The figure shows three views and two pictorial views of one solid part (mm, origin at its lowest corner). Answer the questions. A direction names the side the tool comes from. Coordinates: 2 decimals unless noted, no trailing zeros. Write each loop counter-clockwise with the first axis right and the second up, starting at its lowest first coordinate (ties: lowest second). Pieces come first, ordered by that corner, then holes. Notation, with made-up numbers: (0.25, 51.5) - (35.25, 51.5) arc R21 cw to (35.25, 88.5) - close; hole circle Ø9 at (19.25, -27). An arc over 180 degrees is marked (long way). Use a Markdown table: item, result. Add a question column.
(1) The part is cut by section C-C, the plane z = 1.25. State how many separate pieces and enclosed holes the cut face has, then the cut area to 3 significant figures.
(2) The part is cut by section B-B, the plane y = 5. Give the vertices of the cut face in (x, z), then the cut area to 3 significant figures.
(3) Find the intervals of material crossed by line 1 (Y direction, x = 48, z = 2.75); line 2 (X direction, y = 45, z = 2.35); line 3 (X direction, y = 26.5, z = 1.75), in increasing order. Write a range as from..to.
(4) The part is cut by section D-D, the plane x = 48. Give the vertices of the cut face in (y, z), then the cut area to 3 significant figures.
(5) A tool of negligible diameter and unlimited length cuts with its end or side. For the marked faces 1 and 2, from which of +Z, -Z, +X, -X, +Y, -Y can it reach the whole face along a straight path? Write none if from no direction.
(6) Given pin 1 Ø2 at (y, z) = (10, 7) entering from -X; pin 2 Ø3 at (y, z) = (34.5, 7) entering from -X; pin 3 Ø1.8 at (y, z) = (45.5, 7) entering from +X, each flat-ended and moving along its own axis, determine where each tip first touches the part or whether it passes through.
(7) The part is cut by section A-A, the plane x = 23.5. Give the vertices of the cut face in (y, z).
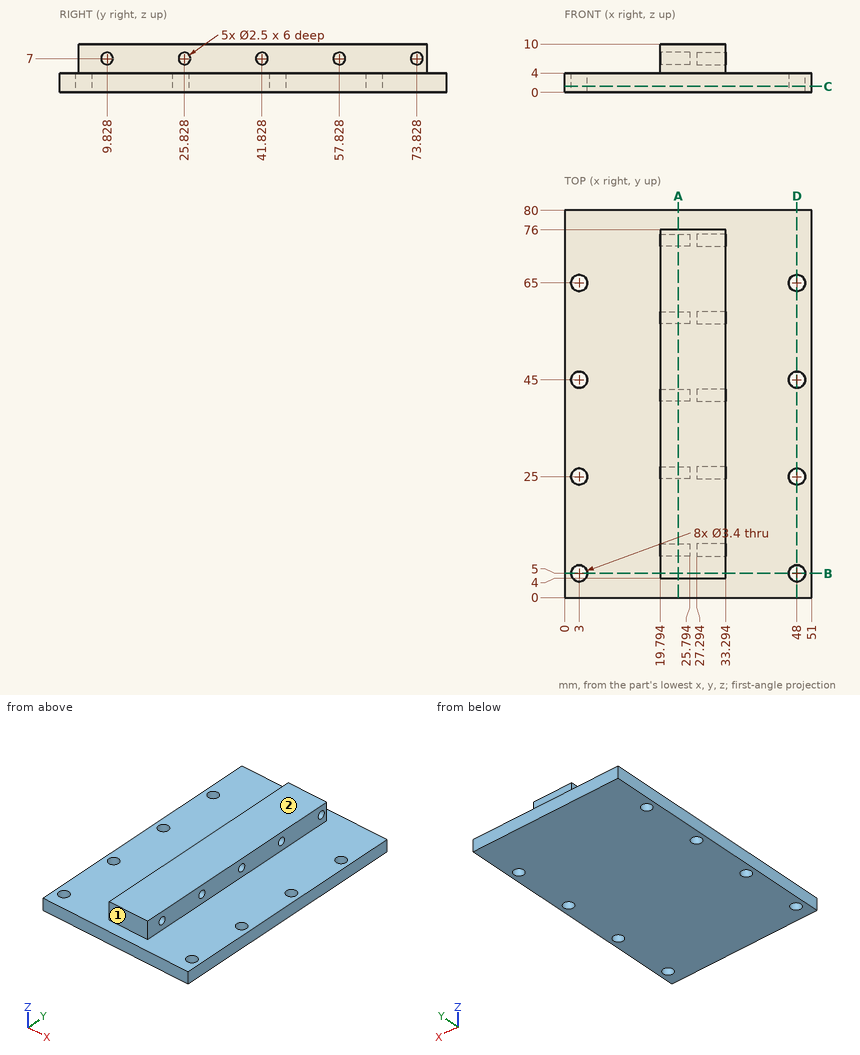
Model answer:
| question | item | result |
|---|---|---|
| 1 | separate pieces | 1 |
| 1 | enclosed holes | 8 |
| 1 | area | 4,010 mm^2 |
| 2 | outline | (0, 0) - (1.3, 0) - (1.3, 4) - (0, 4) - close; (4.7, 0) - (46.3, 0) - (46.3, 4) - (33.29, 4) - (33.29, 10) - (19.79, 10) - (19.79, 4) - (4.7, 4) - close; (49.7, 0) - (51, 0) - (51, 4) - (49.7, 4) - close |
| 2 | area | 258 mm^2 |
| 3 | line 1 | 0..3.3, 6.7..23.3, 26.7..43.3, 46.7..63.3, 66.7..80 |
| 3 | line 2 | 0..1.3, 4.7..46.3, 49.7..51 |
| 3 | line 3 | 0..2.2, 3.8..47.2, 48.8..51 |
| 4 | outline | (0, 0) - (3.3, 0) - (3.3, 4) - (0, 4) - close; (6.7, 0) - (23.3, 0) - (23.3, 4) - (6.7, 4) - close; (26.7, 0) - (43.3, 0) - (43.3, 4) - (26.7, 4) - close; (46.7, 0) - (63.3, 0) - (63.3, 4) - (46.7, 4) - close; (66.7, 0) - (80, 0) - (80, 4) - (66.7, 4) - close |
| 4 | area | 266 mm^2 |
| 5 | face 1 | +Z, +X, -X, -Y |
| 5 | face 2 | +Z, +X, -X, +Y, -Y |
| 6 | pin 1 | x = 25.79 |
| 6 | pin 2 | x = 19.79 |
| 6 | pin 3 | x = 33.29 |
| 7 | outline | (0, 0) - (80, 0) - (80, 4) - (76, 4) - (76, 10) - (4, 10) - (4, 4) - (0, 4) - close; hole circle Ø2.5 at (9.83, 7); hole circle Ø2.5 at (25.83, 7); hole circle Ø2.5 at (41.83, 7); hole circle Ø2.5 at (57.83, 7); hole circle Ø2.5 at (73.83, 7) |
